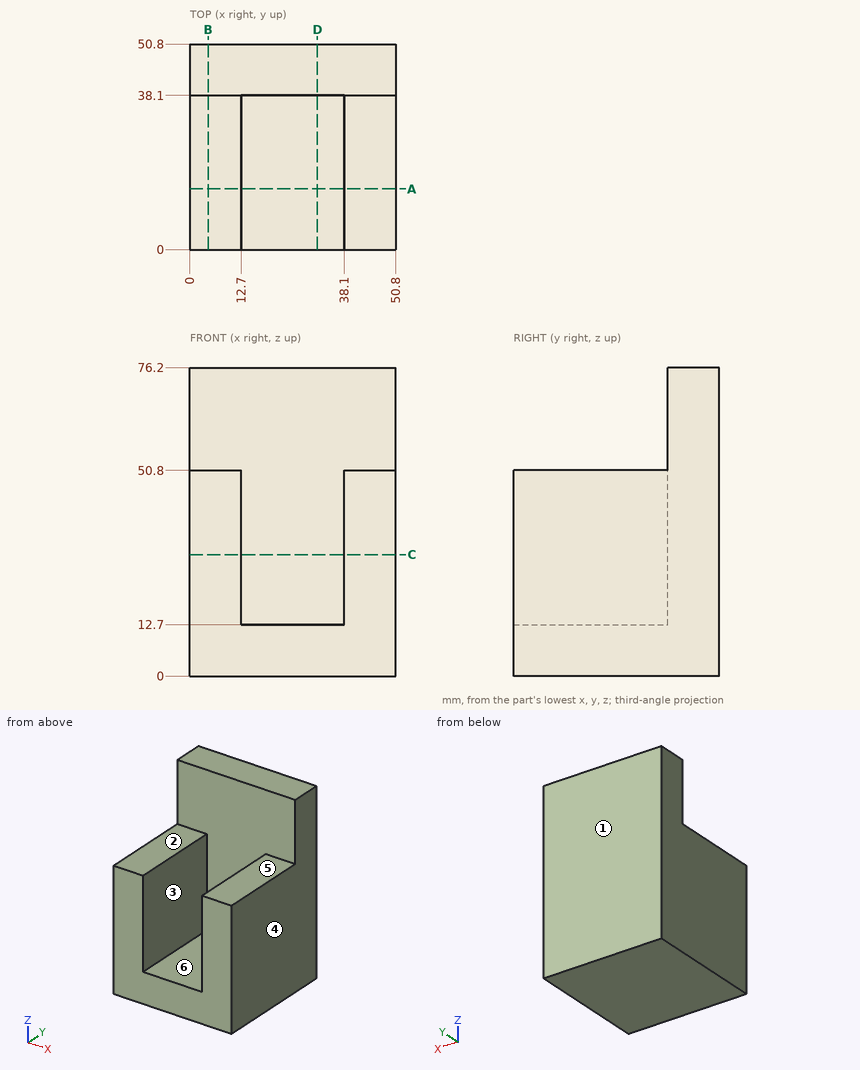
Could you check a few things on this drawing? It's one solid part, dimensions in mm from its lowest x, y, z. A direction names the side the tool comes from. Round coordinates to 2 decimals unless told otherwise and drop trailing zeros. Write each loop counter-clockwise with the first axis right and the second up, starting at its lowest first coordinate (ties: lowest second). Pieces come first, ordered by that corner, then holes.
Q1. Will these pins go through, and if not, where does the flat tip stop? P1, Ø6.5, axis at x = 46, y = 27, coming from the +Z side; P2, Ø12, axis at x = 28.5, y = 29.5, coming from the +Z side; P3, Ø10, axis at x = 25.5, z = 35.5, coming from the -Y side.
Q2. If we section it at A-A on y = 15: Write out the boundary of the cut face in (x, z), plus the area to 3 significant figures.
Q3. If we mould it in two halves opening along X, with no side actions, what happens to the marked faces 4, 5 and 6? For each: +X half, -X half, draft (parallel to the pull), parting line (faces both ways), or undercut.
Q4. Please list where these lines run through material, in increasing order: probe 1 along X at (y, z) = (23, 23); probe 2 along Y at (x, z) = (16.5, 47); probe 3 along Z at (x, y) = (35, 20).
Q5. If we section it at C-C on z = 30: Write out the boundary of the cut face in (x, y).
Q6. If we section it at B-B on x = 4.5: Write out the boundary of the cut face in (y, z), plus the area to 3 significant figures.
Q7. Which directions (+Z, -Z, +X, -X, +Y, -Y) give clear straight access to the entire face, cutting with the end or side of a thin tool? Please do the marked faces 1, 2 and 3.
Q8. If we section it at D-D on x = 31.5: Write out the boundary of the cut face in (y, z), plus the area to 3 significant figures.
Answer below:
1. P1: stops at z = 50.8
1. P2: stops at z = 12.7
1. P3: stops at y = 38.1
2. outline: (0, 0) - (50.8, 0) - (50.8, 50.8) - (38.1, 50.8) - (38.1, 12.7) - (12.7, 12.7) - (12.7, 50.8) - (0, 50.8) - close
2. area: 1,610 mm2
3. face 4: +X half
3. face 5: draft
3. face 6: undercut
4. probe 1: x = 0 to 12.7, 38.1 to 50.8
4. probe 2: y = 38.1 to 50.8
4. probe 3: z = 0 to 12.7
5. outline: (0, 0) - (12.7, 0) - (12.7, 38.1) - (38.1, 38.1) - (38.1, 0) - (50.8, 0) - (50.8, 50.8) - (0, 50.8) - close
6. outline: (0, 0) - (50.8, 0) - (50.8, 76.2) - (38.1, 76.2) - (38.1, 50.8) - (0, 50.8) - close
6. area: 2,900 mm2
7. face 1: +Z, -Z, +X, -X, +Y
7. face 2: +Z, +X, -X, -Y
7. face 3: +Z, -Y
8. outline: (0, 0) - (50.8, 0) - (50.8, 76.2) - (38.1, 76.2) - (38.1, 12.7) - (0, 12.7) - close
8. area: 1,450 mm2
